from build123d import *

# Parameters (mm, degrees)
SKETCH1_R           = 19.25
BOSS_EXTRUDE1_DEPTH = 1
SKETCH2_R           = 11.25
SKETCH2_R_2         = 10
BOSS_EXTRUDE2_DEPTH = 4
SKETCH3_R           = 19.25
SKETCH3_R_2         = 18.75
BOSS_EXTRUDE3_DEPTH = 4
SKETCH5_R           = 10
CUT_EXTRUDE1_DEPTH  = 5


with BuildPart() as part:
    # Sketch1 → Boss-Extrude1 (new body)
    with BuildSketch(Plane.XY):
        Circle(SKETCH1_R)
    extrude(amount=BOSS_EXTRUDE1_DEPTH)

    # Sketch2 → Boss-Extrude2 (add)
    with BuildSketch(Plane.XY.offset(1)):
        Circle(SKETCH2_R)
        Circle(SKETCH2_R_2, mode=Mode.SUBTRACT)
    extrude(amount=BOSS_EXTRUDE2_DEPTH)

    # Sketch3 → Boss-Extrude3 (add)
    with BuildSketch(Plane.XY.offset(1)):
        Circle(SKETCH3_R)
        Circle(SKETCH3_R_2, mode=Mode.SUBTRACT)
    extrude(amount=BOSS_EXTRUDE3_DEPTH)

    # Sketch5 → Cut-Extrude1 (cut)
    with BuildSketch(Plane.XY.offset(1)):
        Circle(SKETCH5_R)
    extrude(amount=-CUT_EXTRUDE1_DEPTH, mode=Mode.SUBTRACT)


solid = part.part
Read the model definition and answer for the solid it produces. Units are mm, in the model's axes. A direction names the side the tool comes from. Coordinates: 2 decimals unless noted, no trailing zeros. Loops run counter-clockwise (first coordinate to the right, second up) from the corner with the lowest first, then second, coordinate; pieces in that order, holes last. Notation, with made-up numbers: (32, -31.5) -> (65, -31.5) arc R31 cw to (65, -6.5) -> close; hole circle Ø2 at (-24.5, 26.25). An arc over 180 degrees is marked (long way). Answer in a Markdown table with one row per item.
Item 1: A cutting plane is placed at C-C on z = 3.6. Determine the outline of the cut face in (x, y), plus the area to 3 significant figures.
Returned:
| item | result |
|---|---|
| outline | circle Ø38.5 at (0, 0); circle Ø22.5 at (0, 0); hole circle Ø37.5 at (0, 0); hole circle Ø20 at (0, 0) |
| area | 143 mm^2 |
Item 2: A cutting plane is placed at A-A on y = 0. Determine the outline of the cut face in (x, z), plus the area to 3 significant figures.
Returned:
| item | result |
|---|---|
| outline | (-19.25, 0) -> (-10, 0) -> (-10, 5) -> (-11.25, 5) -> (-11.25, 1) -> (-18.75, 1) -> (-18.75, 5) -> (-19.25, 5) -> close; (10, 0) -> (19.25, 0) -> (19.25, 5) -> (18.75, 5) -> (18.75, 1) -> (11.25, 1) -> (11.25, 5) -> (10, 5) -> close |
| area | 32.5 mm^2 |
Item 3: Straight lines are drawn through the part: line 1 along Y through (x, z) = (0, 3); line 2 along Y through (x, z) = (0, 0.3); line 3 along Y through (x, z) = (7, 1.3). For each, find the intervals that lie inside material, in ascending order. Write a range as [from, to].
Returned:
| item | result |
|---|---|
| line 1 | y = [-19.25, -18.75], [-11.25, -10], [10, 11.25], [18.75, 19.25] |
| line 2 | y = [-19.25, -10], [10, 19.25] |
| line 3 | y = [-17.93, -17.39], [-8.81, -7.14], [7.14, 8.81], [17.39, 17.93] |
Item 4: For a pull along X with two mould halves and no side action, classify faces 1 (the cylindrical face through (-15.28, -11.71, 2.46)), 2 (the cylindrical face through (5.19, -9.98, 2.97)), 3 (the flat face through (4.19, -18.45, 5)) as released by +X, released by -X, zero draft, split by the parting line, or undercut.
Returned:
| item | result |
|---|---|
| face 1 | split by the parting line |
| face 2 | undercut |
| face 3 | zero draft |
Item 5: Each of these flat-tipped pins is pushed along its axis until it touches: P1, Ø1, axis at y = 14.5, z = 1, coming from the -X side; P2, Ø2, axis at y = 9.5, z = 1.5, coming from the -X side; P3, Ø1, axis at x = -3, z = 3.5, coming from the +Y side. Where does it stop, or does it pass through?
Returned:
| item | result |
|---|---|
| P1 | stops at x = -13.21 |
| P2 | stops at x = -17.27 |
| P3 | stops at y = 19.09 |
Item 6: For faces 4 (the flat face through (-8, -7, 5)), 5 (the cylindrical face through (-2.44, 18.59, 2.97)), determine the directions among +Z, -Z, +X, -X, +Y, -Y from which every point of the face is accessible in a straight line to the end or side of a thin tool.
Returned:
| item | result |
|---|---|
| face 4 | +Z, +X, -X, +Y, -Y |
| face 5 | +Z |
Item 7: A cutting plane is placed at D-D on x = 12. Determine the outline of the cut face in (y, z), plus the area to 3 significant figures.
Returned:
| item | result |
|---|---|
| outline | (-15.05, 0) -> (15.05, 0) -> (15.05, 5) -> (14.41, 5) -> (14.41, 1) -> (-14.41, 1) -> (-14.41, 5) -> (-15.05, 5) -> close |
| area | 35.3 mm^2 |
